Autodesk Inventor part; units mm, degrees
ref_plane "YZ Plane" through (0, 0, 0) normal (1, 0, 0) x (0, 1, 0)
ref_plane "XZ Plane" through (0, 0, 0) normal (0, 1, 0) x (-1, 0, 0)
ref_plane "XY Plane" through (0, 0, 0) normal (0, 0, 1) x (1, 0, 0)
sketch "Skizze1" plane through (0, 0, 0) normal (0, 0, 1) x (1, 0, 0)
  line L0 (-1.2, -1.2) -> (-1.2, -18.6)
  line L1 (-1.2, -18.6) -> (-28.6, -18.6)
  line L2 (-28.6, -18.6) -> (-28.6, -2.2)
  line L3 (0, 0) -> (0, -19.8)
  line L4 (0, -19.8) -> (-29.8, -19.8)
  line L5 (-29.8, -19.8) -> (-29.8, -3.4)
  line L6 (-29.8, -3.4) -> (-35.8, -3.4)
  line L7 (-35.8, -3.4) -> (-35.8, -2.2)
  line L8 (-35.8, -2.2) -> (-28.6, -2.2)
  line L9 (-1.2, -1.2) -> (-35.8, -1.2)
  line L10 (-35.8, -1.2) -> (-35.8, 0)
  line L11 (-35.8, 0) -> (0, 0)
  line L12 (0, -23.76) -> (0, 3.96)
  line L13 (-42.96, 0) -> (7.16, 0)
  point P0 (7.16, 0)
  dimension "d6" = 17.4
  dimension "d7" = 27.4
  dimension "d8" = 16.4
  dimension "d9" = 90
  dimension "d10" = 6
  dimension "d11" = 90
  dimension "d12" = 1.2
  dimension "d13" = 1.2
  dimension "d14" = 1.2
  dimension "d15" = 1.2
  dimension "d16" = 0
  dimension "d17" = 0
  dimension "d18" = 1.2
extrude "Extrusion1" add sketch "Skizze1" along normal blind 9
sketch "Skizze2" plane through (-35.8, -3.4, 0) normal (0, -1, 0) x (1, 0, 0)
  circle A0 centre (3, 3) radius 1.6
  line L0 (0, 9) -> (6, 9)
  line L1 (0, 0) -> (0, 9)
  line L2 (0, 0) -> (6, 0)
  line L3 (6, 9) -> (0, 9)
  line L4 (0, 9) -> (0, 6)
  line L5 (0, 6) -> (6, 6)
  line L6 (6, 6) -> (6, 9)
  point P0 (35.8, 0)
  dimension "d21" = 3.2
  dimension "d23" = 3
  dimension "d75" = 3
  dimension "d76" = 6
  dimension "d77" = 3
extrude "Extrusion2" cut sketch "Skizze2" against normal through all
sketch "Skizze15" plane through (-29.8, -19.8, 0) normal (-1, 0, 0) x (0, 0, 1)
  line L0 (9, 17.6) -> (9, 0)
  line L1 (9, 0) -> (19, 0)
  line L2 (9, 0) -> (19, 0) construction
  line L3 (19, 0) -> (21.8284, -2.8284)
  line L4 (21.8284, -2.8284) -> (22.677, -1.9799)
  line L5 (9, 1.2) -> (19.4971, 1.2)
  line L6 (19.4971, 1.2) -> (22.677, -1.9799)
  line L7 (6, 19.8) -> (9, 19.8)
  line L8 (9, 19.8) -> (9, 18.6)
  line L9 (9, 19.8) -> (9, 18.6)
  line L10 (9, 19.8) -> (19, 19.8)
  line L11 (9, 19.8) -> (19, 19.8) construction
  line L12 (19, 19.8) -> (26.3, 12.5)
  line L13 (9, 18.6) -> (6, 18.6)
  line L14 (9, 18.6) -> (18.5029, 18.6)
  line L15 (18.5029, 18.6) -> (25.4515, 11.6515)
  line L16 (25.4515, 11.6515) -> (26.3, 12.5)
  line L17 (28.3, -13.6) -> (28.3, -12.6)
  point P0 (0, 19.8)
  dimension "d78" = 10
  dimension "d79" = 0
  dimension "d80" = 4
  dimension "d81" = 135
  dimension "d82" = 1.2
  dimension "d83" = 0
  dimension "d84" = 10
  dimension "d85" = 0
  dimension "d86" = 135
  dimension "d87" = 2
  dimension "d88" = 1.2
extrude "Extrusion8" add sketch "Skizze15" against normal up to surface (29.8 mm away)
sketch "Skizze16" plane through (0, -19.8, 0) normal (1, 0, 0) x (0, 0, -1)
  line L0 (-22.677, -1.9799) -> (-19.4971, 1.2)
  line L1 (-19.4971, 1.2) -> (-9, 1.2)
  line L2 (-9, 1.2) -> (-9, 18.6)
  line L3 (-9, 18.6) -> (-18.5029, 18.6)
  line L4 (-18.5029, 18.6) -> (-25.4515, 11.6515)
  line L5 (-25.4515, 11.6515) -> (-26.3, 12.5)
  line L6 (-25.4515, 11.6515) -> (-26.3, 12.5)
  line L7 (-22.677, -1.9799) -> (-26.3, 12.5)
  point P0 (0, 19.8)
extrude "Extrusion9" add sketch "Skizze16" against normal up to surface (1.2 mm away)
sketch "Skizze17" plane through (-29.8, -19.8, 0) normal (-1, 0, 0) x (0, 0, 1)
  line L0 (9, 17.6) -> (9, 1.2)
  line L1 (9, 1.2) -> (19.4971, 1.2)
  line L2 (19.4971, 1.2) -> (22.677, -1.9799)
  line L3 (25.4515, 11.6515) -> (26.3, 12.5)
  line L4 (18.5029, 18.6) -> (25.4515, 11.6515)
  line L5 (18.5029, 18.6) -> (6, 18.6)
  line L6 (9, 17.6) -> (9, 18.6)
  line L7 (22.677, -1.9799) -> (26.3, 12.5)
  point P0 (0, 19.8)
extrude "Extrusion10" add sketch "Skizze17" against normal up to surface (1.2 mm away)
fillet "Rundung1" radius 10 4 edges at (-14.9, -19.8, 19) (-14.9, 0, 19) (-14.9, -18.6, 19.4971) (-14.9, -1.2, 18.5029)
properties part number "shroud 01 volcano" material "ABS-Kunststoff"
Geometry check sheet. Reference: the model listing, model coordinates, mm. A direction names the side the tool comes from. Coordinates: 2 decimals unless noted, no trailing zeros. Write each loop counter-clockwise with the first axis right and the second up, starting at its lowest first coordinate (ties: lowest second). Pieces come first, ordered by that corner, then holes. Notation, with made-up numbers: M 17,51 L 44,51 A23 ccw 44,66 Z; hole C 60.25,51.5 d4. An arc over 180 degrees is marked long. Answer as a JSON object with one key per item and string values.
1. Tool access check on faces 1 (the cylindrical face through (-15.09, -19.38, 19.23)), 2 (the flat face through (-15, -18.6, 8)), 3 (the flat face through (-34.1, -3.4, 1.6)). Record the directions out of +Z, -Z, +X, -X, +Y, -Y that give a thin tool (end or side, any length) a straight path to the whole face; none if there is none.
Answers below:
{"face 1": "+Z", "face 2": "+Z, -Z", "face 3": "+Z, -Z, -X, -Y"}
2. Go/stop test with flat-tipped pins: pin 1 Ø1 at (x, z) = (-17.5, 4.5) entering from -Y; pin 2 Ø4 at (x, z) = (-22, 17) entering from +Y; pin 3 Ø6 at (x, z) = (-12.5, 23) entering from +Y. Record where each tip stops, or that it passes through.
Answers below:
{"pin 1": "stops at y = -19.8", "pin 2": "stops at y = 0", "pin 3": "stops at y = -1.42"}
3. Section check B-B, the plane z = 3. Enter the section's corners in (x, y), plus the area to 3 significant figures.
Answers below:
{"outline": "M -35.8,-3.4 L -34.4,-3.4 L -34.4,-2.2 L -35.8,-2.2 Z; M -35.8,-1.2 L -34.4,-1.2 L -34.4,0 L -35.8,0 Z; M -31.2,-3.4 L -29.8,-3.4 L -29.8,-19.8 L 0,-19.8 L 0,0 L -31.2,0 L -31.2,-1.2 L -1.2,-1.2 L -1.2,-18.6 L -28.6,-18.6 L -28.6,-2.2 L -31.2,-2.2 Z", "area": "119 mm²"}
4. Draft check along X on faces 4 (the flat face through (-15, -5, 24)), 5 (the cylindrical face through (-34.4, -0.61, 3.07)), 6 (the cylindrical face through (-15.092, -1.982, 18.238)), 7 (the flat face through (-35.8, -1, 3)). Enter one of: released by +X, released by -X, zero draft, split by the parting line, or undercut.
Answers below:
{"face 4": "zero draft", "face 5": "undercut", "face 6": "undercut", "face 7": "released by -X"}
5. Scan lines: L1, parallel to X at y = -15.5, z = 5.25; L2, parallel to Y at x = -28.5, z = 13.5; L3, parallel to Z at x = -32.8, y = -0.55. Record each from-to range of solid material in increasing order.
Answers below:
{"L1": "x = -29.8 to -28.6, -1.2 to 0", "L2": "y = -19.8 to -18.6, -1.2 to 0", "L3": "z = 0 to 1.4, 4.6 to 6"}
6. Section check D-D, the plane y = -11.5. Enter the section's corners in (x, z).
Answers below:
{"outline": "M -29.8,0 L -28.6,0 L -28.6,25.25 L -29.8,25.25 Z; M -1.2,0 L 0,0 L 0,25.25 L -1.2,25.25 Z"}
7. Section check C-C, the plane z = 11. Enter the section's corners in (x, y), plus the area to 3 significant figures.
Answers below:
{"outline": "M -29.8,-19.8 L 0,-19.8 L 0,0 L -29.8,0 Z; hole M -28.6,-18.6 L -1.2,-18.6 L -1.2,-1.2 L -28.6,-1.2 Z", "area": "113 mm²"}
8. Section check A-A, the plane x = -12.5. Enter the section's corners in (y, z), plus the area to 3 significant figures.
Answers below:
{"outline": "M -22.63,21.83 A10 cw -19.8,14.86 L -19.8,0 L -18.6,0 L -18.6,15.35 A10 ccw -21.53,22.43 L -21.78,22.68 Z; M -8.15,25.45 L -4.13,21.43 A10 cw -1.2,14.36 L -1.2,0 L 0,0 L 0,14.86 A10 ccw -2.93,21.93 L -7.3,26.3 Z", "area": "62.8 mm²"}
